Answer from the drawing. Dimensions are ordinates in mm from the lowest x, y and z of the part. Round coordinates to 2 decimals unless told otherwise and drop trailing zeros. Loops run counter-clockwise (first coordinate to the right, second up) from the corner with the lowest first, then second, coordinate; pieces in that order, holes last.
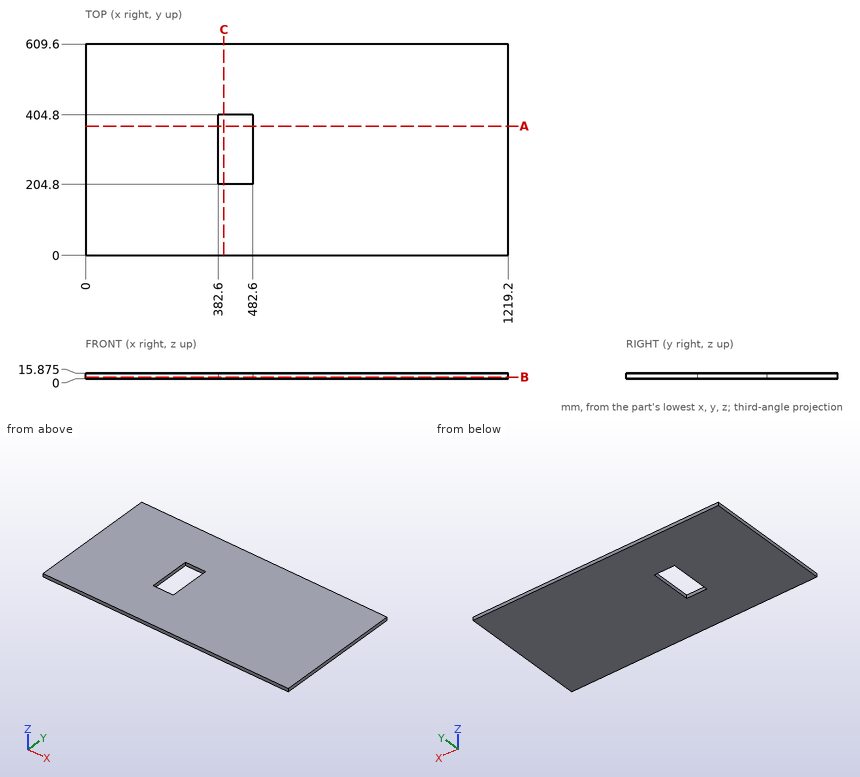
Item 1: Section C-C, the plane x = 399 is taken. Give the vertices of the cut face in (y, z) (3 decimals).
Item 2: A straight line is drawn through the part: line 1 (X direction, y = 281, z = 6.5). Find the intervals that lie inside material, in ascending order.
Item 3: Section B-B, the plane z = 5 is taken. Give the vertices of the cut face in (x, y), plus the area to 3 significant figures.
Item 4: Section A-A, the plane y = 372.5 is taken. Give the vertices of the cut face in (x, z) (3 decimals).
Answer below:
1. outline: (0, 0) - (204.8, 0) - (204.8, 15.875) - (0, 15.875) - close; (404.8, 0) - (609.6, 0) - (609.6, 15.875) - (404.8, 15.875) - close
2. line 1: x = 0 to 382.6, 482.6 to 1219.2
3. outline: (0, 0) - (1219.2, 0) - (1219.2, 609.6) - (0, 609.6) - close; hole (382.6, 204.8) - (482.6, 204.8) - (482.6, 404.8) - (382.6, 404.8) - close
3. area: 723,000 mm2
4. outline: (0, 0) - (382.6, 0) - (382.6, 15.875) - (0, 15.875) - close; (482.6, 0) - (1219.2, 0) - (1219.2, 15.875) - (482.6, 15.875) - close
